Autodesk Inventor part; units mm, degrees
ref_plane "YZ Plane" through (0, 0, 0) normal (1, 0, 0) x (0, 1, 0)
ref_plane "XZ Plane" through (0, 0, 0) normal (0, 1, 0) x (-1, 0, 0)
ref_plane "XY Plane" through (0, 0, 0) normal (0, 0, 1) x (1, 0, 0)
sketch "Sketch1" plane through (0, 0, 0) normal (0, 0, 1) x (1, 0, 0)
  line L0 (0, 0) -> (114, 0)
  line L1 (114, 0) -> (114, 25)
  line L2 (114, 25) -> (0, 25)
  line L3 (0, 25) -> (0, 0)
  dimension "d0" = 25
  dimension "d1" = 114
extrude "Extrusion1" add sketch "Sketch1" against normal blind 12.5
fillet "Fillet1" radius 12.5 2 edges at (57, 25, -12.5) (57, 0, -12.5)
sketch "Sketch2" plane through (0, 0, 0) normal (0, 0, 1) x (1, 0, 0)
  line L0 (114, 0) -> (114, 25)
  line L1 (114, 25) -> (0, 25)
  line L2 (0, 25) -> (0, 0)
  line L3 (0, 0) -> (114, 0)
extrude "Extrusion2" add sketch "Sketch2" along normal blind 1
fillet "Fillet2" radius 3 2 edges at (0, 12.5, 1) (114, 12.5, 1)
sketch "Sketch3" plane through (0, 0, 1) normal (0, 0, 1) x (1, 0, 0)
  circle A0 centre (12.38, 6) radius 1.6
  circle A1 centre (12.38, 19) radius 1.6
  circle A2 centre (40.88, 12.5) radius 1.6
  circle A3 centre (72.88, 12.5) radius 1.6
  circle A4 centre (101.38, 6) radius 1.6
  circle A5 centre (101.38, 19) radius 1.6
  circle A6 centre (12.38, 19) radius 2.15
  circle A7 centre (12.38, 6) radius 2.15
  circle A8 centre (40.88, 12.5) radius 2.15
  circle A9 centre (72.88, 12.5) radius 2.15
  circle A10 centre (101.38, 19) radius 2.15
  circle A11 centre (101.38, 6) radius 2.15
  line L0 (3, 0) -> (111, 0)
  line L1 (111, 25) -> (3, 25)
  circle A12 centre (12.38, 12.5) radius 2.15
  circle A13 centre (100.7971, 12.5) radius 2.15
  point P0 (0, 0)
  dimension "d8" = 4.3
  dimension "d9" = 4.3
  dimension "d10" = 4.3
  dimension "d11" = 4.3
  dimension "d12" = 4.3
  dimension "d13" = 4.3
  dimension "d16" = 25
  dimension "d17" = 4.3
  dimension "d18" = 12.5
  dimension "d19" = 4.3
extrude "Extrusion3" cut sketch "Sketch3" against normal blind 6 contours A12 | A13
equation "\"d9\" = d8"
equation "\"d10\" = d8"
equation "\"d11\" = d8"
equation "\"d12\" = d8"
equation "\"d13\" = d8"
equation "\"d17\" = d8"
equation "\"d18\" = 0.5 * d16"
properties part number "handle_insert"
The listing builds one solid part. Answer for the finished solid, in the listing's coordinates (mm). A direction names the side the tool comes from. Round coordinates to 2 decimals unless told otherwise and drop trailing zeros. Write each loop counter-clockwise with the first axis right and the second up, starting at its lowest first coordinate (ties: lowest second). Pieces come first, ordered by that corner, then holes. Notation, with made-up numbers: (-27, 69) - (19, 69) arc R31 ccw to (19, 93) - close; hole circle Ø7 at (47, -30.5). An arc over 180 degrees is marked (long way). Use one line per item in the form item = value. Start each with the question number.
Item 1: A cutting plane is placed at B-B (y = 18.75). Write down the section's boundary in (x, z), plus the area to 3 significant figures.
Item 2: A cutting plane is placed at D-D (z = -7.75). Write down the section's boundary in (x, y), plus the area to 3 significant figures.
Item 3: Determine the mould class of faces 3 (the cylindrical face through (102.848, 13.146, -1.958)), 4 (the cylindrical face through (113.1, 12.68, 0.14)), 5 (the flat face through (0, 13, -6)) for opening direction X: +X half, -X half, draft (parallel to the pull), parting line (faces both ways), or undercut.
Item 4: A tool of negligible diameter and unlimited length cuts with its end or side. For faces 1 (the cylindrical face through (13.37, 10.59, -1.96)), 2 (the cylindrical face through (0.9, 12.32, 0.14)), from which of +Z, -Z, +X, -X, +Y, -Y can it reach the whole face along a straight path? Write none if from no direction.
Item 5: Flat-ended cylindrical pins translate along their axes: pin 1 Ø1.5 at (x, y) = (82, 11) entering from -Z; pin 2 Ø4 at (x, y) = (12.38, 12.5) entering from +Z; pin 3 Ø12 at (x, y) = (32, 22.5) entering from -Z. Find the tip coordinate at first contact, or state that the pin passes through.
Item 6: Find the intervals of material crossed by line 1 (Y direction, x = 79.5, z = -2); line 2 (Z direction, x = 84.5, y = 16.25); line 3 (Z direction, x = 33.5, y = 7.5), in increasing order. Write a range as [from, to].
The answers:
q1.outline = (0, -10.83) - (114, -10.83) - (114, -2) arc R3 ccw to (111, 1) - (3, 1) arc R3 ccw to (0, -2) - close
q1.area = 1,340 mm^2
q2.outline = (0, 2.69) - (114, 2.69) - (114, 22.31) - (0, 22.31) - close
q2.area = 2,240 mm^2
q3.face_3 = undercut
q3.face_4 = +X half
q3.face_5 = -X half
q4.face_1 = +Z
q4.face_2 = +Z, -X, +Y, -Y
q5.pin_1 = -12.48
q5.pin_2 = -5
q5.pin_3 = -11.84
q6.line_1 = [0.16, 24.84]
q6.line_2 = [-11.92, 1]
q6.line_3 = [-11.46, 1]
